Drawing for the job (mm, zero at the part's lowest x, y, z). A direction names the side the tool comes from. Round coordinates to 2 decimals unless told otherwise and drop trailing zeros. Order: outer loops, then holes, each group sorted by start corner. A loop starts at its lowest first (then second) coordinate and runs counter-clockwise, first axis right, second up. Notation, with made-up numbers: (-30.75, 81) - (24.25, 81) arc R22 cw to (24.25, 94) - close; hole circle Ø7 at (-39.75, 33). An arc over 180 degrees is marked (long way). Put each result on its own line as item: value. Start each with the question number.
Item 1: Probe probe 1 along Y at (x, z) = (32.8, 27.5); probe 2 along Z at (x, y) = (33, 17) (1 decimal); probe 3 along Z at (x, y) = (33, 36.5) (1 decimal). List the from-to ranges inside material, lowest first.
Item 2: Saw through at C-C on x = 11.5. List the corners of the cut face in (y, z).
Item 3: Saw through at B-B on y = 27.5. List the corners of the cut face in (x, z), plus the area to 3 significant figures.
Item 4: Saw through at A-A on y = 6.86. List the corners of the cut face in (x, z).
Item 5: Saw through at D-D on y = 37. State how many separate pieces and enclosed holes the cut face has.
Item 6: Pin check, flat tips, straight feed: pin 1 Ø3 at (x, y) = (14.5, 33) entering from -Z; pin 2 Ø12 at (y, z) = (20, 18) entering from -X; pin 3 Ø3 at (x, y) = (25, 28.5) entering from -Z; pin 4 Ø4 at (x, z) = (21, 42) entering from -Y. Stop position of each tip, or through.
Item 7: Which spindle directions (+Z, -Z, +X, -X, +Y, -Y) get a long thin tool onto all of the face, cutting with end or side? Do the marked faces 1 and 2. Say none if no direction does.
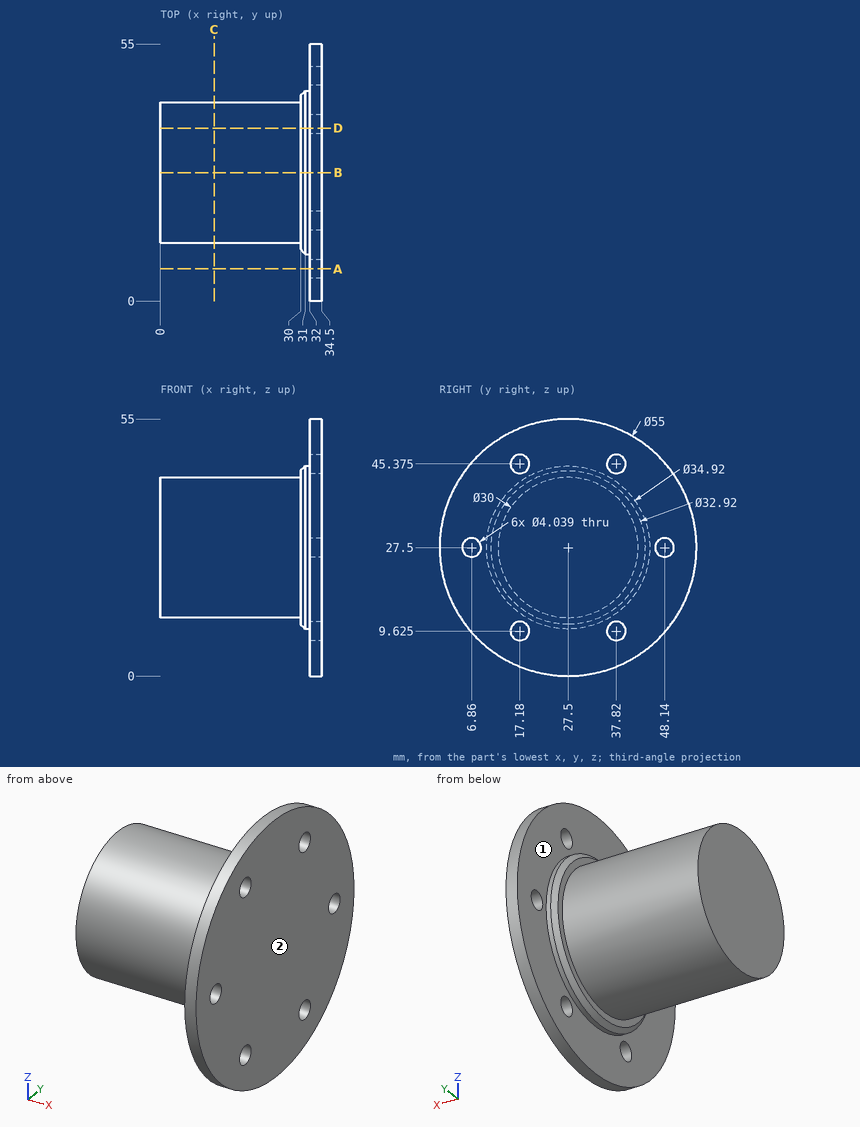
Results found:
1. probe 1: y = 0 to 4.84, 8.88 to 46.12, 50.16 to 55
1. probe 2: z = 2.1 to 7.6, 11.6 to 43.4, 47.4 to 52.9
1. probe 3: z = 1.5 to 8.1, 11.2 to 43.8, 46.9 to 53.5
2. outline: circle Ø30 at (27.5, 27.5)
3. outline: (0, 12.5) - (30, 12.5) - (30, 11.04) - (31, 10.04) - (32, 10.04) - (32, 0) - (34.5, 0) - (34.5, 55) - (32, 55) - (32, 44.96) - (31, 44.96) - (30, 43.96) - (30, 42.5) - (0, 42.5) - close
3. area: 1,110 mm²
4. outline: (32, 9.33) - (34.5, 9.33) - (34.5, 25.48) - (32, 25.48) - close; (32, 29.52) - (34.5, 29.52) - (34.5, 45.67) - (32, 45.67) - close
5. separate pieces: 3
5. enclosed holes: 0
6. pin 1: stops at z = 13.04
6. pin 2: stops at x = 0
6. pin 3: stops at z = 12.5
6. pin 4: stops at y = 19.21
7. face 1: -X
7. face 2: +Z, -Z, +X, +Y, -Y
